Work out the finished part from the listing and answer in its coordinate system (mm). Face numbers are marked on the shaded views. A direction names the side the tool comes from. Coordinates: 2 decimals unless noted, no trailing zeros. Order: outer loops, then holes, each group sorted by start corner. A loop starts at its lowest first (then second) coordinate and runs counter-clockwise, first axis right, second up. Notation, with made-up numbers: M 3.25,-19 L 40.25,-19 A14 cw 40.25,-8 Z; hole C 34,49 d10. An arc over 180 degrees is marked long. Answer in a Markdown table with one row per item. Add a question column.
Item 1: Flat-ended cylindrical pins translate along their axes: pin 1 Ø12 at (x, y) = (44.5, -49) entering from -Z; pin 2 Ø0.9 at (x, y) = (-2.5, -60.5) entering from -Z; pin 3 Ø0.8 at (x, y) = (72.5, 2.5) entering from -Z. Find the tip coordinate at first contact, or state that the pin passes through.
Item 2: The mould has two halves that part along Y. Classify the marked faces 1, 2 and 3: released by +Y, released by -Y, zero draft, split by the parting line, or undercut.
Item 3: Consider line 1 (X direction, y = -26, z = 3.5); line 2 (Y direction, x = 20, z = 4.25); line 3 (Z direction, x = 77, y = -35). Determine where each line is inside the solid, lowest interval first. Write a range as from..to.
Item 4: The part is cut by section A-A (z = 7.25). Write down the section's boundary in (x, y).
Item 5: The part is cut by section C-C (y = -2.5). Write down the section's boundary in (x, z), then the cut area to 3 significant figures.
Item 6: The part is cut by section B-B (x = 15). Write down the section's boundary in (y, z), then the cut area to 3 significant figures.
Item 7: Which of the six approach directions +Z, -Z, +X, -X, +Y, -Y give full straight-line access (tool end or side, diameter ignored) to the marked faces 4 and 5?
Item 8: The part is cut by section D-D (x = 81). Write down the section's boundary in (y, z), then the cut area to 3 significant figures.
from build123d import *

# Parameters (mm, degrees)
SKETCH033_W     = 119.5
SKETCH033_H     = 76
SKETCH033_W_2   = 105.5
SKETCH033_H_2   = 62
PAD011_DEPTH    = 20
SKETCH034_W     = 119.5
SKETCH034_H     = 76
PAD012_DEPTH    = 7
SKETCH035_W     = 12.399995
SKETCH035_H     = 14
POCKET012_DEPTH = 7
CHAMFER_SIZE    = 6
FILLET_R        = 7
SKETCH037_R     = 1.45
POCKET013_DEPTH = 15
CHAMFER006_SIZE = 3


with BuildPart() as part:
    # Sketch033 (on Face1 of Binder012) → Pad011 (new body)
    with BuildSketch(Plane.XY.offset(-1.6)):
        with Locations((50.75, -29)):
            Rectangle(SKETCH033_W, SKETCH033_H)
        with Locations((50.75, -29)):
            Rectangle(SKETCH033_W_2, SKETCH033_H_2, mode=Mode.SUBTRACT)
    extrude(amount=PAD011_DEPTH)

    # Sketch034 (on Face10 of Pad011) → Pad012 (join)
    with BuildSketch(Plane.XY.offset(18.4)):
        with Locations((50.75, -29)):
            Rectangle(SKETCH034_W, SKETCH034_H)
    extrude(amount=PAD012_DEPTH)

    # Sketch035 (on Face9 of Pad012) → Pocket012 (cut)
    with BuildSketch(Plane(origin=(0, 9, 0), x_dir=(-1, 0, 0), z_dir=(0, 1, 0))):
        with Locations((-70.371465, 5.4)):
            Rectangle(SKETCH035_W, SKETCH035_H)
    extrude(amount=-POCKET012_DEPTH, mode=Mode.SUBTRACT)

    # Chamfer
    chamfer_edges = [part.edges().sort_by_distance(p)[0] for p in [
        (70.371465, 9, 12.4),
        (64.171468, 9, 5.4),
        (76.571463, 9, 5.4),
    ]]
    chamfer(chamfer_edges, length=CHAMFER_SIZE)

    # Fillet
    fillet_edges = [part.edges().sort_by_distance(p)[0] for p in [
        (103.5, 2, 8.4),
        (-2, 2, 8.4),
        (-2, -60, 8.4),
        (103.5, -60, 8.4),
    ]]
    fillet(fillet_edges, radius=FILLET_R)

    # Sketch037 (on Face1 of Fillet) → Pocket013 (cut)
    with BuildSketch(Plane(origin=(0, 0, -1.6), x_dir=(1, 0, 0), z_dir=(0, 0, -1))):
        with Locations((-2, 60)):
            Circle(SKETCH037_R)
        with Locations((103.5, 60)):
            Circle(SKETCH037_R)
        with Locations((103.5, -2)):
            Circle(SKETCH037_R)
        with Locations((-2, -2)):
            Circle(SKETCH037_R)
    extrude(amount=-POCKET013_DEPTH, mode=Mode.SUBTRACT)

    # Chamfer006
    chamfer006_edges = [part.edges().sort_by_distance(p)[0] for p in [
        (110.5, 9, 11.9),
        (50.75, 9, 25.4),
        (110.5, -29, 25.4),
        (110.5, -67, 11.9),
        (50.75, -67, 25.4),
        (-9, 9, 11.9),
        (-9, -29, 25.4),
        (-9, -67, 11.9),
    ]]
    chamfer(chamfer006_edges, length=CHAMFER006_SIZE)


solid = part.part
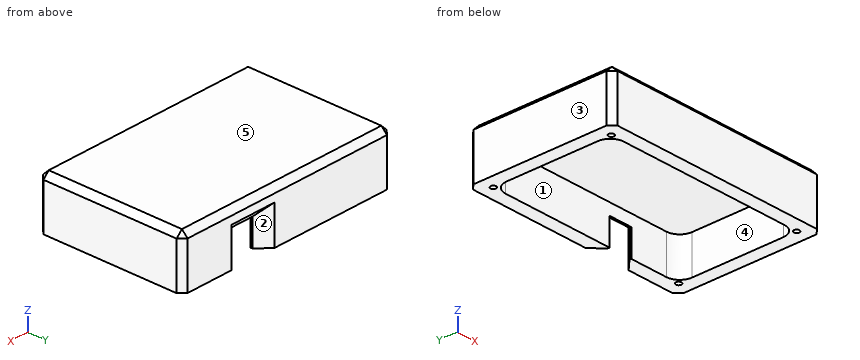
Reply:
| question | item | result |
|---|---|---|
| 1 | pin 1 | stops at z = 18.4 |
| 1 | pin 2 | stops at z = 13.4 |
| 1 | pin 3 | stops at z = 12.4 |
| 2 | face 1 | undercut |
| 2 | face 2 | released by +Y |
| 2 | face 3 | zero draft |
| 3 | line 1 | x = -9..-2, 103.5..110.5 |
| 3 | line 2 | y = -67..-60, 2..9 |
| 3 | line 3 | z = 18.4..25.4 |
| 4 | outline | M -9,-64 L -6,-67 L 107.5,-67 L 110.5,-64 L 110.5,6 L 107.5,9 L 82.57,9 L 76.57,3 L 76.57,2 L 96.5,2 A7 cw 103.5,-5 L 103.5,-53 A7 cw 96.5,-60 L 5,-60 A7 cw -2,-53 L -2,-5 A7 cw 5,2 L 64.17,2 L 64.17,3 L 58.17,9 L -6,9 L -9,6 Z; hole C -2,-60 d2.9; hole C -2,2 d2.9; hole C 103.5,-60 d2.9; hole C 103.5,2 d2.9 |
| 5 | outline | M -9,-1.6 L -1.54,-1.6 L -1.54,18.4 L 103.04,18.4 L 103.04,-1.6 L 110.5,-1.6 L 110.5,22.4 L 107.5,25.4 L -6,25.4 L -9,22.4 Z |
| 5 | area | 1,130 mm2 |
| 6 | outline | M -67,-1.6 L -60,-1.6 L -60,18.4 L 2,18.4 L 2,-1.6 L 9,-1.6 L 9,22.4 L 6,25.4 L -64,25.4 L -67,22.4 Z |
| 6 | area | 803 mm2 |
| 7 | face 4 | -Z |
| 7 | face 5 | +Z, +X, -X, +Y, -Y |
| 8 | outline | M -67,-1.6 L -60,-1.6 L -60,18.4 L 2,18.4 L 2,-1.6 L 7.43,-1.6 L 7.43,16.83 L 9,18.4 L 9,22.4 L 6,25.4 L -64,25.4 L -67,22.4 Z |
| 8 | area | 773 mm2 |
